from build123d import *

# Parameters (mm, degrees)
F0_R     = 3.5
F1_DEPTH = 1


with BuildPart() as f1:
    # F0 (on Front) → F1 (new body)
    with BuildSketch(Plane.XZ):
        Polygon((-61.145082, 190), (-61.145082, 0), (433.854918, 0), (433.854918, 190), (393.854918, 190), (393.854918, 310), (186.354918, 310), (-21.145082, 310), (-21.145082, 190), align=None)
        with Locations((-43.645082, 17)):
            Circle(F0_R, mode=Mode.SUBTRACT)
        with Locations((186.354918, 17)):
            Circle(F0_R, mode=Mode.SUBTRACT)
        with Locations((416.354918, 17)):
            Circle(F0_R, mode=Mode.SUBTRACT)
        with Locations((-43.645082, 167)):
            Circle(F0_R, mode=Mode.SUBTRACT)
        with Locations((76.354918, 297)):
            Circle(F0_R, mode=Mode.SUBTRACT)
        with Locations((416.354918, 167)):
            Circle(F0_R, mode=Mode.SUBTRACT)
        with Locations((296.354918, 297)):
            Circle(F0_R, mode=Mode.SUBTRACT)
    extrude(amount=F1_DEPTH)


solid = f1.part
The model under review builds one solid part; all positions refer to its coordinate system, in mm. Give positions to 0.01 mm unless a question says otherwise; leave off trailing zeros. Order: outer loops, then holes, each group sorted by start corner. A loop starts at its lowest first (then second) coordinate and runs counter-clockwise, first axis right, second up. Notation, with made-up numbers: (68, 41) -> (80, 41) arc R33 cw to (80, 75) -> close; hole circle Ø7 at (43, 89). An arc over 180 degrees is marked (long way). Write item = value, one per line. Start each with the question number.
(1) Take a section at A-A (y = -0.65). Write out the cut boundary in (x, z).
(2) For L1, parallel to X at y = -0.55, z = 167; L2, parallel to X at y = -0.8, z = 297; L3, parallel to Z at x = 394, y = -0.15, list the stretches that pass through material, from the lowest coordinate up. Write a range as from..to.
(3) Take a section at B-B (x = -28.5). Write out the cut boundary in (y, z).
(4) For pin 1 Ø9 at (x, z) = (296.35, 297) entering from -Y; pin 2 Ø0.5 at (y, z) = (-0.5, 256) entering from -X, all flat-tipped, find the tip position at first contact; note any pin that passes through.
Returned:
q1.outline = (-61.15, 0) -> (433.85, 0) -> (433.85, 190) -> (393.85, 190) -> (393.85, 310) -> (-21.15, 310) -> (-21.15, 190) -> (-61.15, 190) -> close; hole circle Ø7 at (-43.65, 17); hole circle Ø7 at (-43.65, 167); hole circle Ø7 at (76.35, 297); hole circle Ø7 at (186.35, 17); hole circle Ø7 at (296.35, 297); hole circle Ø7 at (416.35, 17); hole circle Ø7 at (416.35, 167)
q2.L1 = -61.15..-47.15, -40.15..412.85, 419.85..433.85
q2.L2 = -21.15..72.85, 79.85..292.85, 299.85..393.85
q2.L3 = 0..190
q3.outline = (-1, 0) -> (0, 0) -> (0, 190) -> (-1, 190) -> close
q4.pin_1 = -1
q4.pin_2 = -21.15
